```python
from build123d import *

# Parameters (mm, degrees)
SKETCH1_W                      = 863.6
SKETCH1_H                      = 63.5
BASE_FLANGE1_DEPTH             = 2.032
EDGE_FLANGE1_STRIP_W           = 14.478
EDGE_FLANGE1_STRIP_H           = 2.032
EDGE_FLANGE1_STRIP_CUT_DEPTH   = 863.6
EDGE_FLANGE1_STRIP_2_W         = 14.478
EDGE_FLANGE1_STRIP_2_H         = 2.032
EDGE_FLANGE1_STRIP_CUT_2_DEPTH = 863.6
EDGE_FLANGE1_DEPTH             = 863.6
EDGE_FLANGE1_BEND_DEPTH        = 863.6


# Sheet-metal steps are written as plain solids
with BuildPart() as part:
    # Sketch1 → Base-Flange1 (new body)
    with BuildSketch(Plane(origin=(0, 0, 0), x_dir=(1, 0, 0), z_dir=(0, 1, 0))):
        with Locations((431.8, 31.75)):
            Rectangle(SKETCH1_W, SKETCH1_H)
    extrude(amount=-BASE_FLANGE1_DEPTH)

    # Edge-Flange1 strip (across the edge) → Edge-Flange1 strip cut (cut)
    with BuildSketch(Plane(origin=(863.6, -2.032, 0), x_dir=(0, 0, -1), z_dir=(-1, 0, 0))):
        with Locations((-2.032, -1.016)):
            Rectangle(EDGE_FLANGE1_STRIP_W, EDGE_FLANGE1_STRIP_H)
    extrude(amount=EDGE_FLANGE1_STRIP_CUT_DEPTH, mode=Mode.SUBTRACT)

    # Edge-Flange1 strip 2 (across the edge) → Edge-Flange1 strip cut 2 (cut)
    with BuildSketch(Plane(origin=(0, -2.032, -63.5), x_dir=(0, 0, 1), z_dir=(1, 0, 0))):
        with Locations((-2.032, -1.016)):
            Rectangle(EDGE_FLANGE1_STRIP_2_W, EDGE_FLANGE1_STRIP_2_H)
    extrude(amount=EDGE_FLANGE1_STRIP_CUT_2_DEPTH, mode=Mode.SUBTRACT)

    # Edge-Flange1 section (across the edge) → Edge-Flange1 (add)
    with BuildSketch(Plane(origin=(863.6, -2.032, 0), x_dir=(0, 0, -1), z_dir=(-1, 0, 0))):
        with BuildLine():
            Line((0, 3.175), (0, 23.368))
            Line((0, 23.368), (2.032, 23.368))
            Line((2.032, 23.368), (2.032, 3.175))
            ThreePointArc((2.032, 3.175), (2.96193597, 0.92993597), (5.207, 0))
            Line((5.207, 0), (5.207, -2.032))
            ThreePointArc((5.207, -2.032), (1.52509499, -0.50690501), (0, 3.175))
        make_face()
    extrude(amount=EDGE_FLANGE1_DEPTH)

    # Edge-Flange1 section 2 (across the edge) → Edge-Flange1 bend (add)
    with BuildSketch(Plane(origin=(0, -2.032, -63.5), x_dir=(0, 0, 1), z_dir=(1, 0, 0))):
        with BuildLine():
            Line((0, 3.175), (0, 23.368))
            Line((0, 23.368), (2.032, 23.368))
            Line((2.032, 23.368), (2.032, 3.175))
            ThreePointArc((2.032, 3.175), (2.96193597, 0.92993597), (5.207, 0))
            Line((5.207, 0), (5.207, -2.032))
            ThreePointArc((5.207, -2.032), (1.52509499, -0.50690501), (0, 3.175))
        make_face()
    extrude(amount=EDGE_FLANGE1_BEND_DEPTH)


solid = part.part
```
CAD build for the part. Positions are in the model's coordinates, mm. A direction names the side the tool comes from. Give positions to 0.01 mm unless a question says otherwise; leave off trailing zeros. Write each loop counter-clockwise with the first axis right and the second up, starting at its lowest first coordinate (ties: lowest second). Pieces come first, ordered by that corner, then holes. Notation, with made-up numbers: M 13,55.25 L 31,55.25 A30 cw 31,78.25 Z; hole C -37.75,78 d11. An arc over 180 degrees is marked long. Return JSON: item names as keys, results as strings. Group by question number.
(1) Mould opens along Z. For faces 3 (the face through (426, -15, -63.5)), 4 (the face through (438, -15, 0)), 5 (the face through (438, -15, -2.032)) say: pulls with the +Z half, pulls with the -Z half, needs draft (parallel to the pull), parting line crosses it, or undercut.
(2) Band-saw the part on A-A (y = -13.25). Give the cut face in (x, z), and give its area (3 significant figures).
(3) 3-axis set-ups, long thin cutter, end or side, ignore diameter. For faces 1 (the face through (0, -1, -32)), 2 (the face through (426, -2.032, -32)): which of +Z, -Z, +X, -X, +Y, -Y reach the whole face in a straight line?
(4) Band-saw the part on B-B (x = 259). Give the cut face in (y, z) (3 decimals).
(5) Drill centre lines: L1, parallel to Z at x = 443.5, y = -24; L2, parallel to Y at x = 382, z = -26.5; L3, parallel to Z at x = 91, y = -1.75. Where is each one in solid material? Low to high. Write a range as [from, to].
(6) Band-saw the part on C-C (z = -18.5). Give the cut face in (x, y), and give its area (3 significant figures).
(7) Flat gauge pins, fed straight in: pin 1 Ø8 at (y, z) = (-4.5, -29) entering from +X; pin 2 Ø5 at (x, z) = (100.5, -39) entering from -Y. Where does each tip first touch, or does it go through?
Entries:
{
 "1": {"face 3": "pulls with the -Z half", "face 4": "pulls with the +Z half", "face 5": "undercut"},
 "2": {"outline": "M 0,-63.5 L 863.6,-63.5 L 863.6,-61.47 L 0,-61.47 Z; M 0,-2.03 L 863.6,-2.03 L 863.6,0 L 0,0 Z", "area": "3,510 mm^2"},
 "3": {"face 1": "+Z, -Z, -X, +Y, -Y", "face 2": "+X, -X, -Y"},
 "4": {"outline": "M -25.4,-63.5 L -5.207,-63.5 A5.207 ccw 0,-58.293 L 0,-5.207 A5.207 ccw -5.207,0 L -25.4,0 L -25.4,-2.032 L -5.207,-2.032 A3.175 cw -2.032,-5.207 L -2.032,-58.293 A3.175 cw -5.207,-61.468 L -25.4,-61.468 Z"},
 "5": {"L1": "z = [-63.5, -61.47], [-2.03, 0]", "L2": "y = [-2.03, 0]", "L3": "z = [-62.19, -1.31]"},
 "6": {"outline": "M 0,-2.03 L 863.6,-2.03 L 863.6,0 L 0,0 Z", "area": "1,750 mm^2"},
 "7": {"pin 1": "stops at x = 863.6", "pin 2": "stops at y = -2.03"}
}
